Here's how the part is built. I have some questions about the finished solid (model axes, mm). A direction names the side the tool comes from. Round coordinates to 2 decimals unless told otherwise and drop trailing zeros. Write each loop counter-clockwise with the first axis right and the second up, starting at its lowest first coordinate (ties: lowest second). Pieces come first, ordered by that corner, then holes. Notation, with made-up numbers: M 2.5,-4.75 L 19.5,-4.75 A24 ccw 19.5,28.25 Z; hole C 14,52 d9. An arc over 180 degrees is marked long. Use one line per item in the form item = value. Start each with the question number.
Q1. I want a section at A-A on z = -5.5. List the corners of the cut face in (x, y) for me (3 decimals), and give its area (3 significant figures).
Q2. For faces 1 (the face through (30, 0, 0)), 2 (the face through (36.87, 3.96, 0.28)), which set-ups out of +Z, -Z, +X, -X, +Y, -Y let a thin tool reach every point of the face, with its end or its side?
Q3. I want a section at C-C on x = 37.75. List the corners of the cut face in (y, z) for me, and give its area (3 significant figures).
Q4. I need wall thicknesses on line 1 along Y through (x, z) = (36, 13.5); line 2 along Y through (x, z) = (37.5, 0). Which ranges of each line are inside material? Lowest first, please. Write a range as from..to.
Q5. We'd pull the mould along Z, two halves only. Please class faces 3 (the face through (40.49, 3.96, 0.28)), 4 (the face through (30, 2, 25)), 5 (the face through (44.775, 2, 0)): +Z half, -Z half, draft (parallel to the pull), parting line (faces both ways), or undercut.
Q6. I want a section at B-B on y = 4.5. List the corners of the cut face in (x, z) for me (3 decimals).
Q7. I'm going to push a flat-ended pin straight in: pin 1 Ø5 at (x, z) = (36.5, -19.5) entering from +Y. Where does the tip first touch, or does it pass through?
```python
from build123d import *

# Parameters (mm, degrees)
SKETCH_1_W          = 89.55
SKETCH_1_H          = 50
EXTRUDE_1_DEPTH     = 5
CUT_EXTRUDE_1_DEPTH = 4
SKETCH_6_W          = 40.5
SKETCH_6_H          = 93
CUT_EXTRUDE_2_DEPTH = 3.43
SKETCH_7_W          = 59.55
SKETCH_7_H          = 5
CUT_EXTRUDE_3_DEPTH = 51


with BuildPart() as part:
    # 草圖1 → 填料-伸長1 (new body)
    with BuildSketch(Plane(origin=(0, 0, 0), x_dir=(1, 0, 0), z_dir=(0, 1, 0))):
        Rectangle(SKETCH_1_W, SKETCH_1_H)
    extrude(amount=EXTRUDE_1_DEPTH)

    # 草圖2 → 除料-伸長1 (cut)
    with BuildSketch(Plane(origin=(0, 5, 0), x_dir=(1, 0, 0), z_dir=(0, 1, 0))):
        Polygon((-39.775, 5.2), (-7.375, 5.2), (-7.375, -5.2), (-39.775, -5.2), (-39.775, -4), (-44.775, -4), (-44.775, 4), (-39.775, 4), align=None)
    extrude(amount=-CUT_EXTRUDE_1_DEPTH, mode=Mode.SUBTRACT)

    # 草圖6 → 除料-伸長2 (cut)
    with BuildSketch(Plane(origin=(5.745095169, 17.681584822, 0), x_dir=(0, 0, -1), z_dir=(0.309016994, 0.951056516, 0))):
        with Locations((0, 9.21448352)):
            Rectangle(SKETCH_6_W, SKETCH_6_H)
    extrude(amount=-CUT_EXTRUDE_2_DEPTH, mode=Mode.SUBTRACT)

    # 草圖7 → 除料-伸長3 (cut, through all)
    with BuildSketch(Plane.XY.offset(25)):
        with Locations((-15, 2.5)):
            Rectangle(SKETCH_7_W, SKETCH_7_H)
    extrude(amount=-CUT_EXTRUDE_3_DEPTH, mode=Mode.SUBTRACT)


solid = part.part
```
Reported:
q1.outline = M 14.775,0 L 44.775,0 L 44.775,5 L 40.829,5 L 40.146,2.898 L 33.675,5 L 14.775,5 Z
q1.area = 142 mm^2
q2.face_1 = +Z, -Z, +X, -X, -Y
q2.face_2 = +Y
q3.outline = M 0,-25 L 5,-25 L 5,-20.25 L 3.68,-20.25 L 3.68,20.25 L 5,20.25 L 5,25 L 0,25 Z
q3.area = 196 mm^2
q4.line_1 = 0..4.24
q4.line_2 = 0..3.76
q5.face_3 = undercut
q5.face_4 = +Z half
q5.face_5 = draft
q6.outline = M 14.775,-25 L 44.775,-25 L 44.775,25 L 14.775,25 Z; hole M 35.214,-20.25 L 40.666,-20.25 L 40.666,20.25 L 35.214,20.25 Z
q7.pin_1 = 5
